Autodesk Inventor part; units mm, degrees
ref_plane "YZ Plane" through (0, 0, 0) normal (1, 0, 0) x (0, 1, 0)
ref_plane "XZ Plane" through (0, 0, 0) normal (0, 1, 0) x (-1, 0, 0)
ref_plane "XY Plane" through (0, 0, 0) normal (0, 0, 1) x (1, 0, 0)
sketch "Sketch1" plane through (0, 0, 0) normal (0, 0, 1) x (1, 0, 0)
  circle A0 centre (0, 0) radius 44.45
  circle A1 centre (0, 0) radius 34.925
  dimension "d0" = 88.9
  dimension "d20" = 69.85
extrude "Extrusion1" add sketch "Sketch1" against normal blind 6.35
sketch "Sketch3" plane through (0, 0, 0) normal (0, 0, 1) x (1, 0, 0)
  circle A0 centre (0, 0) radius 41.402 construction
  line L0 (0, 0) -> (29.2756, 29.2756) construction
  circle A1 centre (0, 0) radius 44.45 construction
  line L1 (-44.45, 0) -> (44.45, 0) construction
  point P0 (-29.2756, 29.2756)
  point P1 (-29.2756, -29.2756)
  point P2 (29.2756, -29.2756)
  dimension "d4" = 82.804
  dimension "d5" = 45
  dimension "d8" = 360
hole "Hole1" at (29.2756, 29.2756, 0) at (-29.2756, 29.2756, 0) at (-29.2756, -29.2756, 0) at (29.2756, -29.2756, 0) direction (0, 0, -1) diameter 3.9624 end through all
sketch "Sketch7" plane through (0, 0, 0) normal (0, 0, 1) x (1, 0, 0)
  circle A0 centre (0, 0) radius 34.925
  circle A1 centre (0, 0) radius 47.625
  dimension "d25" = 95.25
extrude "Extrusion4" add sketch "Sketch7" along normal blind 3.175
sketch "Sketch8" plane through (0, 0, 3.175) normal (0, 0, 1) x (1, 0, 0)
  circle A0 centre (0, 0) radius 40.64 construction
  point P0 (40.64, 0)
  point P1 (0, 40.64)
  point P2 (-40.64, 0)
  point P3 (0, -40.64)
  dimension "d28" = 81.28
  dimension "d38" = 360
hole "Hole2" at (0, 40.64, 3.175) at (-40.64, 0, 3.175) at (0, -40.64, 3.175) at (40.64, 0, 3.175) direction (0, 0, -1) diameter 5.1054 end through all
properties part number "LS-002" material "Aluminum 6061"
Design review of the part built by this model. Coordinates are the model's own, in mm. A direction names the side the tool comes from. Coordinates: 2 decimals unless noted, no trailing zeros. Order: outer loops, then holes, each group sorted by start corner. A loop starts at its lowest first (then second) coordinate and runs counter-clockwise, first axis right, second up.
1) Mouldability with a two-part tool opening along X and no side actions: class faces 3 (the flat face through (29, -29, 0)), 4 (the cylindrical face through (42.397, 13.352, -3.131)), 5 (the flat face through (20, -29, -6.35)) as +X half, -X half, draft (parallel to the pull), parting line (faces both ways), or undercut.
2) Wall thickness on line 1 along Y through (x, z) = (-1, 2); line 2 along X through (y, z) = (-4.5, -2); line 3 along Y through (x, z) = (15, 0.5): over which ranges is each line inside the solid? List them lowest first.
3) Take a section at A-A, the plane x = 0. Give the boundary of the cut face in (y, z) (3 decimals).
4) Take a section at C-C, the plane y = 21.5. Give the boundary of the cut face in (x, z) (3 decimals), and give its area (3 significant figures).
5) For faces 1 (the flat face through (29, 29, 0)), 2 (the flat face through (-25, 25, 3.175)), list the 3-axis set-ups (+Z, -Z, +X, -X, +Y, -Y) from which the entire face can be reached by the end or side of a thin tool; tool diameter is ignored.
6) Take a section at D-D, the plane x = 24.5. Give the boundary of the cut face in (y, z) (3 decimals), and give its area (3 significant figures).
7) Clearance check with flat-ended pins moving along their axes: pin 1 (3 mm diameter, centred on y = 17.5, z = -2, fed in from -X); pin 2 (1.2 mm diameter, centred on x = 29.5, y = 29.5, fed in from -Z); pin 3 (4 mm diameter, centred on x = -40.64, y = 0, fed in from -Z); pin 4 (1.5 mm diameter, centred on x = -1, z = 1.5, fed in from -Y). State where each tip first meets the part, or that it passes through.
Returned:
1. face 3: undercut
1. face 4: parting line
1. face 5: draft
2. line 1: y = -47.61 to -42.99, -38.29 to -34.91, 34.91 to 38.29, 42.99 to 47.61
2. line 2: x = -44.22 to -34.63, 34.63 to 44.22
2. line 3: y = -45.2 to -31.54, 31.54 to 45.2
3. outline: (-47.625, 0) - (-44.45, 0) - (-44.45, -6.35) - (-43.193, -6.35) - (-43.193, 3.175) - (-47.625, 3.175) - close; (-38.087, -6.35) - (-34.925, -6.35) - (-34.925, 3.175) - (-38.087, 3.175) - close; (34.925, -6.35) - (38.087, -6.35) - (38.087, 3.175) - (34.925, 3.175) - close; (43.193, -6.35) - (44.45, -6.35) - (44.45, 0) - (47.625, 0) - (47.625, 3.175) - (43.193, 3.175) - close
4. outline: (-42.496, 0) - (-38.904, 0) - (-38.904, -6.35) - (-27.523, -6.35) - (-27.523, 3.175) - (-42.496, 3.175) - close; (27.523, -6.35) - (38.904, -6.35) - (38.904, 0) - (42.496, 0) - (42.496, 3.175) - (27.523, 3.175) - close
4. area: 240 mm2
5. face 1: -Z
5. face 2: +Z, +X, -X, +Y, -Y
6. outline: (-40.84, 0) - (-37.088, 0) - (-37.088, -6.35) - (-24.89, -6.35) - (-24.89, 3.175) - (-40.84, 3.175) - close; (24.89, -6.35) - (37.088, -6.35) - (37.088, 0) - (40.84, 0) - (40.84, 3.175) - (24.89, 3.175) - close
6. area: 256 mm2
7. pin 1: stops at x = -41.47
7. pin 2: stops at z = 0
7. pin 3: passes through
7. pin 4: stops at y = -47.62
